from build123d import *

# Parameters (mm, degrees)
F0_R     = 8
F1_DEPTH = 1
F4_W     = 5
F4_H     = 5
F5_DEPTH = 25
F6_DEPTH = 26.197


with BuildPart() as f1:
    # F0 (on Top) → F1 (new body)
    with BuildSketch(Plane.XY):
        with BuildLine():
            Line((-73, -42.5), (73, -42.5))
            ThreePointArc((73, -42.5), (77.9497474683, -40.4497474683), (80, -35.5))
            Line((80, -35.5), (80, 35.5))
            ThreePointArc((80, 35.5), (77.9497474683, 40.4497474683), (73, 42.5))
            Line((73, 42.5), (-73, 42.5))
            ThreePointArc((-73, 42.5), (-77.9497474683, 40.4497474683), (-80, 35.5))
            Line((-80, 35.5), (-80, -35.5))
            ThreePointArc((-80, -35.5), (-77.9497474683, -40.4497474683), (-73, -42.5))
        make_face()
        Circle(F0_R, mode=Mode.SUBTRACT)
        Circle(F0_R)
    extrude(amount=F1_DEPTH)

    # F4 (on face) → F5 (cut)
    with BuildSketch(Plane(origin=(0, 0, 0), x_dir=(1, 0, 0), z_dir=(0, 0, -1))):
        Rectangle(F4_W, F4_H)
    extrude(amount=-F5_DEPTH, mode=Mode.SUBTRACT)

    # F3 (on face) → F6 (join)
    with BuildSketch(Plane(origin=(0, 0, 0), x_dir=(1, 0, 0), z_dir=(0, 0, -1))):
        with BuildLine():
            ThreePointArc((-7.8251753865, 1.6633190224), (0, 8), (7.8251753865, 1.6633190224))
            Line((7.8251753865, 1.6633190224), (5.3723529412, 25))
            Line((5.3723529412, 25), (-5.3723529412, 25))
            Line((-5.3723529412, 25), (-7.8251753865, 1.6633190224))
        make_face()
        with BuildLine():
            Line((6.4233442804, -15), (7.8251605833, -1.6633886632))
            ThreePointArc((7.8251605833, -1.6633886632), (-3.55984e-05, -7.9999999999), (-7.8251753865, -1.6633190224))
            Line((-7.8251753865, -1.6633190224), (-6.4234117647, -15))
            Line((-6.4234117647, -15), (3.0757090009, -15))
            Line((3.0757090009, -15), (6.4233442804, -15))
        make_face()
        Polygon((-5.3723529412, 25), (5.3723529412, 25), (4.0585294118, 37.5), (-4.0585294118, 37.5), align=None)
        Polygon((4.0583607009, -37.5), (6.4233442804, -15), (3.0757090009, -15), (-6.4234117647, -15), (-4.0585294118, -37.5), align=None)
    extrude(amount=F6_DEPTH)


solid = f1.part
For this review, take the finished solid that the model builds, in its own axes (mm). A direction names the side the tool comes from. Give positions to 0.01 mm unless a question says otherwise; leave off trailing zeros. Loops run counter-clockwise (first coordinate to the right, second up) from the corner with the lowest first, then second, coordinate; pieces in that order, holes last. Notation, with made-up numbers: M -12,51 L 7,51 A19 cw 7,57 Z; hole C 25,82.25 d11. An arc over 180 degrees is marked long. Put each result on its own line as item: value. Start each with the question number.
(1) Wall thickness on L1, parallel to Y at x = 0, z = -4; L2, parallel to Z at x = -16.5, y = -36.5; L3, parallel to Y at x = -2, z = -2.75: over which ranges is each line inside the solid? List them lowest first.
(2) Add section C-C, the plane x = 23.5. Write out the cut boundary in (y, z).
(3) Add section A-A, the plane z = -10.75. Write out the cut boundary in (x, y).
(4) For pin 1 (12 mm diameter, centred on x = -18.5, y = 7, fed in from -Z); pin 2 (1 mm diameter, centred on y = -20, z = -9.5, fed in from +X); pin 3 (9 mm diameter, centred on x = -2, z = -16.5, fed in from +Y), all flat-tipped, find the tip position at first contact; note any pin that passes through.
(5) Add section B-B, the plane y = 17.5. Write out the cut boundary in (x, z), then the cut area to 3 significant figures.
(6) Add section D-D, the plane y = 31. Write out the cut boundary in (x, z).
(7) Machinability: for faces 1 (the flat face through (-5.915, -19.833, -12.915)), 2 (the flat face through (0, -37.5, -13)), 3 (the cylindrical face through (0, -8, -13)), 4 (the flat face through (0, 37.5, -13)), which of the approach directions +Z, -Z, +X, -X, +Y, -Y give a long, thin tool a straight path to every point of the face, cutting with its end or side? Answer none if there is none.
Result:
1. L1: y = -37.5 to -8, 8 to 37.5
1. L2: z = 0 to 1
1. L3: y = -37.5 to -7.75, 7.75 to 37.5
2. outline: M -42.5,0 L 42.5,0 L 42.5,1 L -42.5,1 Z
3. outline: M -7.83,-1.66 L -4.06,-37.5 L 4.06,-37.5 L 7.83,-1.66 A8 cw Z; M -7.83,1.66 A8 cw 7.83,1.66 L 4.06,37.5 L -4.06,37.5 Z
4. pin 1: stops at z = 0
4. pin 2: stops at x = 5.95
4. pin 3: stops at y = 37.5
5. outline: M -80,0 L -6.16,0 L -6.16,-26.2 L 6.16,-26.2 L 6.16,0 L 80,0 L 80,1 L -80,1 Z
5. area: 483 mm^2
6. outline: M -80,0 L -4.74,0 L -4.74,-26.2 L 4.74,-26.2 L 4.74,0 L 80,0 L 80,1 L -80,1 Z
7. face 1: -Z, -X, -Y
7. face 2: -Z, +X, -X, -Y
7. face 3: -Z
7. face 4: -Z, +X, -X, +Y
